The listing builds one solid part. Answer for the finished solid, in the listing's coordinates (mm). A direction names the side the tool comes from. Coordinates: 2 decimals unless noted, no trailing zeros. Order: outer loops, then holes, each group sorted by start corner. A loop starts at its lowest first (then second) coordinate and runs counter-clockwise, first axis right, second up. Notation, with made-up numbers: (11.25, -6.5) -> (30.25, -6.5) arc R20 cw to (30.25, 29.5) -> close; hole circle Ø3 at (83, 74). An arc over 180 degrees is marked (long way). One line per question, with ' | ' between items.
from build123d import *

# Parameters (mm, degrees)
SKETCH_1_R             = 16
EXTRUDE_1_DEPTH        = 8
FILLET_1_R             = 2
SKETCH_4_R             = 16
SKETCH_4_R_2           = 12.5
EXTRUDE_2_DEPTH        = 3
HOLE_WIZARD_M4_3_D     = 3.3
HOLE_WIZARD_M4_3_DEPTH = 6
HOLE_WIZARD_M4_4_D     = 3.3
HOLE_WIZARD_M4_4_DEPTH = 6


with BuildPart() as part:
    # 草图1 → 凸台-拉伸1 (new body)
    with BuildSketch(Plane.XY):
        with BuildLine():
            Line((-26, 23.6), (26, 23.6))
            Line((26, 23.6), (26, 17.6))
            Line((26, 17.6), (9.49947367, 17.6))
            ThreePointArc((9.49947367, 17.6), (19.423244762, 4.76839207), (16.569852142, -11.2))
            Line((16.569852142, -11.2), (26, -11.2))
            Line((26, -11.2), (26, -17.2))
            Line((26, -17.2), (-26, -17.2))
            Line((-26, -17.2), (-26, -11.2))
            Line((-26, -11.2), (-16.569852142, -11.2))
            ThreePointArc((-16.569852142, -11.2), (-19.423244762, 4.76839207), (-9.49947367, 17.6))
            Line((-9.49947367, 17.6), (-26, 17.6))
            Line((-26, 17.6), (-26, 23.6))
        make_face()
        Circle(SKETCH_1_R, mode=Mode.SUBTRACT)
    extrude(amount=EXTRUDE_1_DEPTH)

    # 圆角1
    fillet_1_edges = [part.edges().sort_by_distance(p)[0] for p in [
        (-26, -11.2, 4),
        (-9.49947367, 17.6, 4),
        (-26, 17.6, 4),
        (26, 17.6, 4),
        (9.49947367, 17.6, 4),
        (26, -11.2, 4),
    ]]
    fillet(fillet_1_edges, radius=FILLET_1_R)

    # 草图4 → 凸台-拉伸2 (add)
    with BuildSketch(Plane(origin=(0, 0, 0), x_dir=(-1, 0, 0), z_dir=(0, 0, -1))):
        Circle(SKETCH_4_R)
        Circle(SKETCH_4_R_2, mode=Mode.SUBTRACT)
    extrude(amount=-EXTRUDE_2_DEPTH)

    # M4 螺纹孔3
    with Locations(Plane(origin=(0, 23.6, 0), x_dir=(1, 0, 0), z_dir=(0, 1, 0))):
        with Locations((20, -4), (-20, -4)):
            Hole(HOLE_WIZARD_M4_3_D / 2, depth=HOLE_WIZARD_M4_3_DEPTH)

    # M4 螺纹孔4
    with Locations(Plane.XZ.offset(17.2)):
        with Locations((20, 4), (-20, 4)):
            Hole(HOLE_WIZARD_M4_4_D / 2, depth=HOLE_WIZARD_M4_4_DEPTH)


solid = part.part
Item 1: Determine the mould class of faces 6 (the face through (25.43, 18.2, 4.06)), 7 (the face through (0, 17, 8)), 8 (the face through (21.31, -14.16, 3)) for opening direction Z: pulls with the +Z half, pulls with the -Z half, needs draft (parallel to the pull), parting line crosses it, or undercut.
Computed values:
face 6: needs draft | face 7: pulls with the +Z half | face 8: undercut
Item 2: Section B-B, the plane z = 6.25 is taken. Give the vertices of the cut face in (x, y), plus the area to 3 significant figures.
Computed values:
outline: (-26, -17.2) -> (26, -17.2) -> (26, -13.2) arc R2 ccw to (24, -11.2) -> (16.57, -11.2) arc R20 ccw to (14.1, 14.18) arc R2 cw to (15.51, 17.6) -> (24, 17.6) arc R2 ccw to (26, 19.6) -> (26, 23.6) -> (-26, 23.6) -> (-26, 19.6) arc R2 ccw to (-24, 17.6) -> (-15.51, 17.6) arc R2 cw to (-14.1, 14.18) arc R20 ccw to (-16.57, -11.2) -> (-24, -11.2) arc R2 ccw to (-26, -13.2) -> close; hole circle Ø32 at (0, 0) | area: 850 mm^2
Item 3: Section D-D, the plane x = 21 is taken. Give the vertices of the cut face in (y, z), plus the area to 3 significant figures.
Computed values:
outline: (-17.2, 0) -> (-11.2, 0) -> (-11.2, 2.69) -> (-17.2, 2.69) -> close; (-17.2, 5.31) -> (-11.2, 5.31) -> (-11.2, 8) -> (-17.2, 8) -> close; (17.6, 0) -> (23.6, 0) -> (23.6, 2.69) -> (17.6, 2.69) -> close; (17.6, 5.31) -> (23.6, 5.31) -> (23.6, 8) -> (17.6, 8) -> close | area: 64.5 mm^2
Item 4: Find the intervals of material crossed by L1, parallel to X at y = 21.35, z = 4; L2, parallel to Z at x = 20, y = -12.75; L3, parallel to Y at x = 0, z = 1.7, in increasing order.
Computed values:
L1: x = -26 to -21.65, -18.35 to 18.35, 21.65 to 26 | L2: z = 0 to 2.35, 5.65 to 8 | L3: y = -17.2 to -12.5, 12.5 to 23.6
Item 5: Section C-C, the plane x = 0 is taken. Give the vertices of the cut face in (y, z).
Computed values:
outline: (-17.2, 0) -> (-12.5, 0) -> (-12.5, 3) -> (-16, 3) -> (-16, 8) -> (-17.2, 8) -> close; (12.5, 0) -> (23.6, 0) -> (23.6, 8) -> (16, 8) -> (16, 3) -> (12.5, 3) -> close
Item 6: For faces 1 (the face through (26, 22, 4)), 2 (the face through (-20, 17.6, 6)), 3 (the face through (-11.923, 3.755, 1.479)), 4 (the face through (-18.69, -14.16, 3)), 5 (the face through (-18.69, 20.56, 5)), determine the directions among +Z, -Z, +X, -X, +Y, -Y from which every point of the face is accessible in a straight line to the end or side of a thin tool.
Computed values:
face 1: +Z, -Z, +X, +Y, -Y | face 2: +Z, -Z, -X | face 3: +Z, -Z | face 4: -Y | face 5: +Y
Item 7: Section A-A, the plane y = 0 is taken. Give the vertices of the cut face in (x, z), plus the area to 3 significant figures.
Computed values:
outline: (-20, 0) -> (-12.5, 0) -> (-12.5, 3) -> (-16, 3) -> (-16, 8) -> (-20, 8) -> close; (12.5, 0) -> (20, 0) -> (20, 8) -> (16, 8) -> (16, 3) -> (12.5, 3) -> close | area: 85.0 mm^2
Item 8: Each of these flat-tipped pins is pushed along its axis until it touches: pin 1 Ø19 at (x, y) = (0, 0) entering from +Z; pin 2 Ø1 at (y, z) = (-9, 3) entering from -X; pin 3 Ø3 at (x, z) = (-20, 4) entering from +Y; pin 4 Ø3.5 at (x, z) = (-19, 4.5) entering from +Y. Where does it stop, or does it pass through?
Computed values:
pin 1: passes through | pin 2: stops at x = -18.1 | pin 3: stops at y = 7.6 | pin 4: stops at y = 23.6
